The listing builds one solid part. Answer for the finished solid, in the listing's coordinates (mm). Round coordinates to 2 decimals unless told otherwise and drop trailing zeros. Write each loop counter-clockwise with the first axis right and the second up, starting at its lowest first coordinate (ties: lowest second). Pieces come first, ordered by that corner, then holes.
Item 1: Find section B-B on z = 9.5. Give the number of separate pieces and of enclosed holes in the cut face, then the cut area to 3 significant figures.
Item 2: Find the intervals of material crossed by probe 1 along Y at (x, z) = (-100, 1.2); probe 2 along Y at (x, z) = (70, 6.5); probe 3 along Z at (x, y) = (-26.5, -4.25), in increasing order.
Item 3: Find section D-D on x = -81. Give the vertices of the cut face in (y, z), then the cut area to 3 significant figures.
Item 4: Find section A-A on x = 70. Give the vertices of the cut face in (y, z), then the cut area to 3 significant figures.
Item 5: Find section C-C on x = 100. Give the vertices of the cut face in (y, z), then the cut area to 3 significant figures.
Item 6: Each of these flat-tipped pins is pushed along its axis until it touches: pin 1 (6.5 mm diameter, centred on x = -22, z = 6.5, fed in from -Y); pin 2 (3.5 mm diameter, centred on x = -100, y = 5, fed in from -Z). Where does it stop, or does it pass through?
Autodesk Inventor part; units mm, degrees
ref_plane "YZ Plane" through (0, 0, 0) normal (1, 0, 0) x (0, 1, 0)
ref_plane "XZ Plane" through (0, 0, 0) normal (0, 1, 0) x (-1, 0, 0)
ref_plane "XY Plane" through (0, 0, 0) normal (0, 0, 1) x (1, 0, 0)
sketch "Sketch7" plane through (0, 0, 0) normal (0, 0, 1) x (1, 0, 0)
  line L0 (-110, -10) -> (110, -10)
  line L1 (110, -10) -> (110, 10)
  line L2 (110, 10) -> (-110, 10)
  line L3 (-110, 10) -> (-110, -10)
  line L4 (-110, -10) -> (110, 10) construction
  line L5 (110, -10) -> (-110, 10) construction
  point P0 (0, 0)
  dimension "d27" = 20
  dimension "d28" = 220
extrude "Extrusion6" add sketch "Sketch7" along normal blind 2.8
sketch "Sketch8" plane through (0, 0, 2.8) normal (0, 0, 1) x (1, 0, 0)
  line L0 (-110, 10) -> (-110, -10)
  line L1 (-110, 0) -> (110, 0)
  line L2 (110, 0) -> (110, 10)
  line L3 (110, 10) -> (-110, 10)
  line L4 (-110, 10) -> (-110, 0)
  point P0 (0, 0)
  dimension "d32" = 10
extrude "Extrusion7" add sketch "Sketch8" along normal blind 9.2
sketch "Sketch9" plane through (0, 0, 12) normal (0, 0, 1) x (1, 0, 0)
  circle A0 centre (-70, 5) radius 2.85
  line L0 (0, 14) -> (0, -14)
  circle A1 centre (70, 5) radius 2.85
  line L1 (110, 10) -> (-110, 10)
  point P0 (0, 0)
  dimension "d35" = 5.7
  dimension "d36" = 5
  dimension "d37" = 70
extrude "Extrusion8" cut sketch "Sketch9" against normal through all
fillet "Fillet4" radius 5 6 edges at (-110, 0, 7.4) (-110, 10, 6) (-110, -10, 1.4) (110, -10, 1.4) (110, 0, 7.4) (110, 10, 6)
sketch "Sketch10" plane through (0, 0, 12) normal (0, 0, 1) x (1, 0, 0)
  circle A0 centre (-100, 5) radius 2.3
  circle A1 centre (-70, 5) radius 2.85
  line L0 (105, 10) -> (-105, 10)
  line L1 (0, 14) -> (0, -14)
  circle A2 centre (100, 5) radius 2.3
  point P0 (0, 0)
  dimension "d43" = 4.6
  dimension "d44" = 100
  dimension "d45" = 5
  dimension "d46" = 5
extrude "Extrusion9" cut sketch "Sketch10" against normal through all contours A0 | A2
sketch "Sketch11" plane through (0, 0, 12) normal (0, 0, 1) x (1, 0, 0)
  line L0 (-115, 10) -> (-94, 10)
  line L1 (-94, 10) -> (-94, -3.6473)
  line L2 (-94, -3.6473) -> (-115, -3.6473)
  line L3 (-115, -3.6473) -> (-115, 10)
  line L4 (-110, 5) -> (-110, -5)
  line L5 (-105, 0) -> (105, 0)
  line L6 (105, 10) -> (-105, 10)
  line L7 (0, 14) -> (0, -14)
  line L8 (115, 10) -> (94, 10)
  line L9 (94, 10) -> (94, -3.6473)
  line L10 (94, -3.6473) -> (115, -3.6473)
  line L11 (115, -3.6473) -> (115, 10)
  line L12 (110, 1.6834) -> (110, -5)
  point P0 (0, 0)
  point P1 (-110, 1.6834)
  point P2 (94, 0)
  dimension "d49" = 16
extrude "Extrusion10" cut sketch "Sketch11" against normal up to surface (9.2 mm away) contours L0 L1 L2 L3 | L6 L8 L11 L10 L9
fillet "Fillet6" radius 5 4 edges at (-94, 0, 7.4) (-94, 10, 7.4) (94, 0, 7.4) (94, 10, 7.4)
fillet "Fillet7" radius 1 3 edges at (-92.5357, 1.4643, 2.8) (92.5357, 1.4643, 2.8) (0, 0, 2.8)
equation "\"d46\" = d45"
properties part number "DisplayHolderUpper_3DPrint"
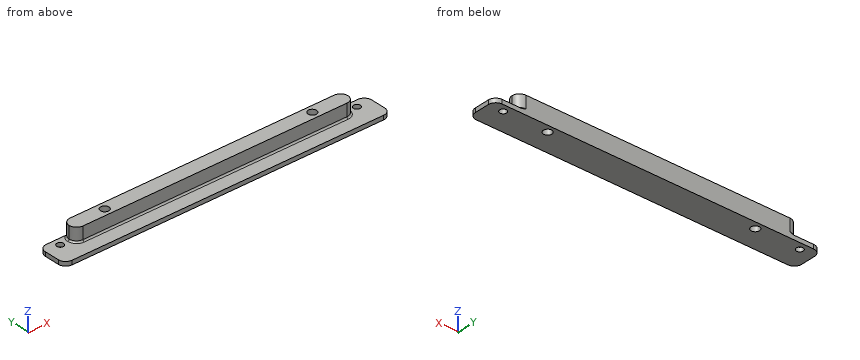
Check values:
1. separate pieces: 1
1. enclosed holes: 2
1. area: 1,810 mm2
2. probe 1: y = -10 to 2.7, 7.3 to 10
2. probe 2: y = 0 to 2.15, 7.85 to 10
2. probe 3: z = 0 to 2.8
3. outline: (-10, 0) - (10, 0) - (10, 12) - (0, 12) - (0, 3.8) arc R1 cw to (-1, 2.8) - (-10, 2.8) - close
3. area: 148 mm2
4. outline: (-10, 0) - (2.15, 0) - (2.15, 12) - (0, 12) - (0, 3.8) arc R1 cw to (-1, 2.8) - (-10, 2.8) - close; (7.85, 0) - (10, 0) - (10, 12) - (7.85, 12) - close
4. area: 79.8 mm2
5. outline: (-10, 0) - (2.7, 0) - (2.7, 2.8) - (-10, 2.8) - close; (7.3, 0) - (10, 0) - (10, 2.8) - (7.3, 2.8) - close
5. area: 43.1 mm2
6. pin 1: stops at y = -0.16
6. pin 2: passes through
